Could you check a few things on this model? Use its own coordinates, in mm. Coordinates: 2 decimals unless noted, no trailing zeros. Write each loop counter-clockwise with the first axis right and the second up, starting at its lowest first coordinate (ties: lowest second). Pieces come first, ordered by that corner, then holes.
```python
from build123d import *

# Parameters (mm, degrees)
CIRPATTERN1_COUNT = 4


with BuildPart() as part:
    # Sketch1 → Revolve2 (revolve)
    with BuildSketch(Plane.XY):
        Polygon((1.5, 0), (1.5, 2.75), (2.938, 2.75), (3, 2.688), (3, 1.312), (2.938, 1.25), (1.875, 1.25), (1.875, 0), align=None)
    revolve(axis=Axis((0, 0, 0), (0, 1, 0)))

    # Sketch4 → Cut-Revolve1 (revolve, cut)
    with BuildSketch(Plane.XY):
        Polygon((-3.475, 2.374), (-2.175, 2.374), (-1.875, 2), (-3.475, 2), align=None)
    cut_revolve1 = revolve(axis=Axis((-3.475, 2, 0), (1, 0, 0)), mode=Mode.SUBTRACT)

    # CirPattern1: Cut-Revolve1 ×4 about axis
    cirpattern1_axis = Axis((0, 2.75, 0), (0, -1, 0))
    for i in range(1, CIRPATTERN1_COUNT):
        add(cut_revolve1.rotate(cirpattern1_axis, i * 360 / CIRPATTERN1_COUNT), mode=Mode.SUBTRACT)


solid = part.part
```
1. Please list where these lines run through material, in increasing order: line 1 along Y through (x, z) = (0, -2.25); line 2 along Y through (x, z) = (-1.5, -2); line 3 along X through (y, z) = (0.3, 0.5).
Verdict:
line 1: y = 1.25 to 1.63, 2.37 to 2.75
line 2: y = 1.25 to 2.75
line 3: x = -1.81 to -1.41, 1.41 to 1.81
2. I want a section at A-A on y = 0.4. Please give me the cut outline in (x, z) (3 decimals).
Verdict:
outline: circle Ø3.75 at (0, 0); hole circle Ø3 at (0, 0)
3. If we mould it in two halves opening along Z, with no side actions, what happens to faces 1 (the face through (2.86, 1.99, -0.9)), 2 (the face through (-1.5, 1.39, -0.07)), 3 (the face through (-1.3, 2.75, 1.3))? For each: pulls with the +Z half, pulls with the -Z half, needs draft (parallel to the pull), parting line crosses it, or undercut.
Verdict:
face 1: parting line crosses it
face 2: undercut
face 3: needs draft
